Check sheet for the drawn part. Datum: minimum x, y, z corner. Units: mm. Coordinates: 2 decimals unless noted, no trailing zeros. Write each loop counter-clockwise with the first axis right and the second up, starting at its lowest first coordinate (ties: lowest second). Pieces come first, ordered by that corner, then holes. Notation, with made-up numbers: (63.25, -15) - (70.25, -15) arc R14 ccw to (70.25, -8) - close; hole circle Ø10 at (75, 32.5). An arc over 180 degrees is marked (long way). Answer as CSV lines item,"result". Start each with the question number.
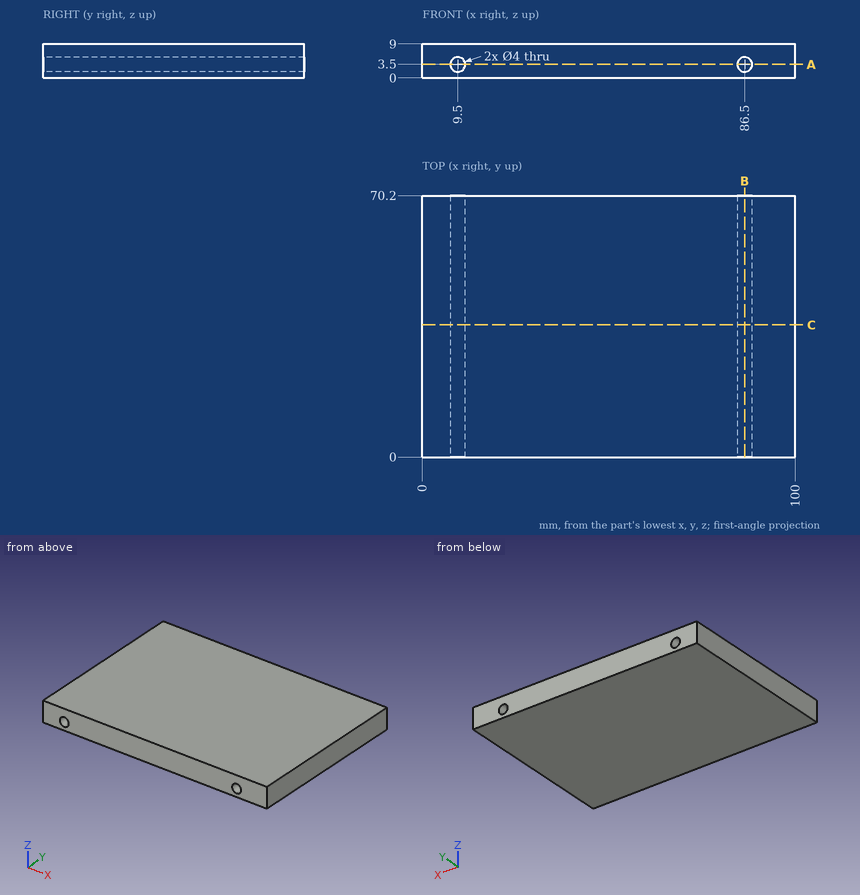
(1) Cross-section at C-C on y = 35.5. Record the boundary of the cut face in (x, z), plus the area to 3 significant figures.
(2) Cross-section at A-A on z = 3.5. Record the boundary of the cut face in (x, y), plus the area to 3 significant figures.
(3) Cross-section at B-B on x = 86.5. Record the boundary of the cut face in (y, z), plus the area to 3 significant figures.
(4) Go/stop test with a flat-tipped pin: P1, Ø3, axis at x = 86.5, z = 3.5, coming from the +Y side. Record where the tip stops, or that it passes through.
(5) Material ranges on probe 1 along X at (y, z) = (63.5, 2.5); probe 2 along X at (y, z) = (27, 5.25); probe 3 along Z at (x, y) = (86, 23), recorded low to high. Write a range as from..to.
Checked values:
1,outline,"(0, 0) - (100, 0) - (100, 9) - (0, 9) - close; hole circle Ø4 at (9.5, 3.5); hole circle Ø4 at (86.5, 3.5)"
1,area,"875 mm^2"
2,outline,"(0, 0) - (7.5, 0) - (7.5, 70.2) - (0, 70.2) - close; (11.5, 0) - (84.5, 0) - (84.5, 70.2) - (11.5, 70.2) - close; (88.5, 0) - (100, 0) - (100, 70.2) - (88.5, 70.2) - close"
2,area,"6,460 mm^2"
3,outline,"(0, 0) - (70.2, 0) - (70.2, 1.5) - (0, 1.5) - close; (0, 5.5) - (70.2, 5.5) - (70.2, 9) - (0, 9) - close"
3,area,"351 mm^2"
4,P1,"through"
5,probe 1,"0..7.77, 11.23..84.77, 88.23..100"
5,probe 2,"0..8.53, 10.47..85.53, 87.47..100"
5,probe 3,"0..1.56, 5.44..9"
